from build123d import *

# Parameters (mm, degrees)
BOSS_EXTRUDE1_DEPTH     = 2.4
BOSS_EXTRUDE2_START     = -2.6
SKETCH2_R               = 0.25
BOSS_EXTRUDE2_DEPTH     = 36.2
CUT_EXTRUDE_THIN1_DEPTH = 0.1


with BuildPart() as part:
    # Sketch1 → Boss-Extrude1 (new body)
    with BuildSketch(Plane(origin=(0, 0, 0), x_dir=(1, 0, 0), z_dir=(0, 1, 0))):
        with BuildLine():
            Line((2.15, 1.37113092), (2.15, -1.37113092))
            ThreePointArc((2.15, -1.37113092), (0, -2.55), (-2.15, -1.37113092))
            Line((-2.15, -1.37113092), (-2.15, 1.37113092))
            ThreePointArc((-2.15, 1.37113092), (0, 2.55), (2.15, 1.37113092))
        make_face()
    extrude(amount=BOSS_EXTRUDE1_DEPTH)

    # Sketch2 → Boss-Extrude2 (add)
    with BuildSketch(Plane.XZ.offset(BOSS_EXTRUDE2_START)):
        with Locations((0, 1.7)):
            Circle(SKETCH2_R)
        with Locations((0, -1.7)):
            Circle(SKETCH2_R)
    extrude(amount=BOSS_EXTRUDE2_DEPTH)

    # Sketch3 → Cut-Extrude-Thin1 (cut)
    with BuildSketch(Plane(origin=(0, 2.4, 0), x_dir=(1, 0, 0), z_dir=(0, 1, 0))):
        with BuildLine():
            ThreePointArc((-2.15, 1.24613092), (-2.021205551, 1.192782512), (-1.967857143, 1.063988063))
            Line((-1.967857143, 1.063988063), (-1.967857143, -0.875))
            ThreePointArc((-1.967857143, -0.875), (-1.535714286, -1.307142857), (-1.103571429, -0.875))
            Line((-1.103571429, -0.875), (-1.103571429, 0.875))
            ThreePointArc((-1.103571429, 0.875), (-0.921428571, 1.057142857), (-0.739285714, 0.875))
            Line((-0.739285714, 0.875), (-0.739285714, -0.875))
            ThreePointArc((-0.739285714, -0.875), (-0.307142857, -1.307142857), (0.125, -0.875))
            Line((0.125, -0.875), (0.125, 0.875))
            ThreePointArc((0.125, 0.875), (0.307142857, 1.057142857), (0.489285714, 0.875))
            Line((0.489285714, 0.875), (0.489285714, -0.875))
            ThreePointArc((0.489285714, -0.875), (0.921428571, -1.307142857), (1.353571429, -0.875))
            Line((1.353571429, -0.875), (1.353571429, 0.875))
            ThreePointArc((1.353571429, 0.875), (1.535714286, 1.057142857), (1.717857143, 0.875))
            Line((1.717857143, 0.875), (1.717857143, -1.063988063))
            ThreePointArc((1.717857143, -1.063988063), (1.844428855, -1.369559208), (2.15, -1.49613092))
            Line((2.15, -1.49613092), (2.15, -1.24613092))
            ThreePointArc((2.15, -1.24613092), (2.021205551, -1.192782512), (1.967857143, -1.063988063))
            Line((1.967857143, -1.063988063), (1.967857143, 0.875))
            ThreePointArc((1.967857143, 0.875), (1.535714286, 1.307142857), (1.103571429, 0.875))
            Line((1.103571429, 0.875), (1.103571429, -0.875))
            ThreePointArc((1.103571429, -0.875), (0.921428571, -1.057142857), (0.739285714, -0.875))
            Line((0.739285714, -0.875), (0.739285714, 0.875))
            ThreePointArc((0.739285714, 0.875), (0.307142857, 1.307142857), (-0.125, 0.875))
            Line((-0.125, 0.875), (-0.125, -0.875))
            ThreePointArc((-0.125, -0.875), (-0.307142857, -1.057142857), (-0.489285714, -0.875))
            Line((-0.489285714, -0.875), (-0.489285714, 0.875))
            ThreePointArc((-0.489285714, 0.875), (-0.921428571, 1.307142857), (-1.353571429, 0.875))
            Line((-1.353571429, 0.875), (-1.353571429, -0.875))
            ThreePointArc((-1.353571429, -0.875), (-1.535714286, -1.057142857), (-1.717857143, -0.875))
            Line((-1.717857143, -0.875), (-1.717857143, 1.063988063))
            ThreePointArc((-1.717857143, 1.063988063), (-1.844428855, 1.369559208), (-2.15, 1.49613092))
            Line((-2.15, 1.49613092), (-2.15, 1.24613092))
        make_face()
    extrude(amount=-CUT_EXTRUDE_THIN1_DEPTH, mode=Mode.SUBTRACT)


solid = part.part
Design review of the part built by this model. Coordinates are the model's own, in mm. Give positions to 0.01 mm unless a question says otherwise; leave off trailing zeros. Loops run counter-clockwise (first coordinate to the right, second up) from the corner with the lowest first, then second, coordinate; pieces in that order, holes last. Notation, with made-up numbers: (83, 48.5) - (132, 48.5) arc R21 ccw to (132, 72.5) - close; hole circle Ø6 at (-6, 0). An arc over 180 degrees is marked (long way). Write item = value, one per line.
1) Clearance check with flat-ended pins moving along their axes: pin 1 Ø1.9 at (x, z) = (0, 0) entering from +Y; pin 2 Ø2 at (x, y) = (0, -10) entering from -Z; pin 3 Ø2 at (y, z) = (-19, 1) entering from -X; pin 4 Ø2 at (x, z) = (-0.5, 1) entering from -Y. State where each tip first meets the part, or that it passes through.
Result sheet:
pin_1 = 2.4
pin_2 = -1.95
pin_3 = -0.25
pin_4 = -33.6
2) To check wall thickness, follow line 1 (Y direction, x = 0.1, z = -1.1); line 2 (Y direction, x = 1.6, z = 1.85); line 3 (Z direction, x = 0.1, y = -17.5). State the ranges of each line that lie inside material, in increasing order.
Result sheet:
line_1 = 0 to 2.3
line_2 = 0 to 2.4
line_3 = -1.93 to -1.47, 1.47 to 1.93
3) Take a section at B-B on y = -5. State the section outline as (x, z) points, and give its area (3 significant figures).
Result sheet:
outline = circle Ø0.5 at (0, -1.7); circle Ø0.5 at (0, 1.7)
area = 0.393 mm2
